Geometry check sheet. Reference: the model listing, model coordinates, mm. A direction names the side the tool comes from. Round coordinates to 2 decimals unless told otherwise and drop trailing zeros. Write each loop counter-clockwise with the first axis right and the second up, starting at its lowest first coordinate (ties: lowest second). Pieces come first, ordered by that corner, then holes. Notation, with made-up numbers: M 47.5,48 L 84.5,48 A23 cw 84.5,60 Z; hole C 30,85.25 d9. An arc over 180 degrees is marked long. One line per item, written item: value. Start each with the question number.
1. Depth check by flat-ended pin: P1, Ø4, axis at x = 9, y = -5.5, coming from the -Z side; P2, Ø2.5, axis at x = 17, y = -5.5, coming from the +Z side; P3, Ø5, axis at y = -4.5, z = -5, coming from the -X side. Enter the tip coordinate at first touch or a pass-through.
2. Scan lines: probe 1 along X at (y, z) = (0.5, -2); probe 2 along Z at (x, y) = (11.5, -6.5); probe 3 along Z at (x, y) = (-3, -7). Record each from-to range of solid material in increasing order. Write a range as [from, to].
3. Release check for a two-part mould opening along X. For faces 4 (the flat face through (19.55, -7, -9)), 5 (the flat face through (13.05, -5, -6)), 6 (the flat face through (18, -7, -7.8)) record: pulls with the +X half, pulls with the -X half, needs draft (parallel to the pull), parting line crosses it, or undercut.
4. Section check D-D (y = -9.5). Record the boundary of the cut face in (x, z).
5. Section check B-B (x = -1.25). Record the boundary of the cut face in (y, z).
6. Access from +Z, -Z, +X, -X, +Y, -Y to the whole of each face (thin tool, end or side, straight path). Record for faces 1 (the flat face through (-2, -2.8, -9)), 2 (the flat face through (1.05, -5, -6)), 3 (the flat face through (16, -5.8, -9)).
7. Section check A-A (z = -9.75). Record the boundary of the cut face in (x, y).
8. Section check C-C (z = -5.25). Record the boundary of the cut face in (x, y).
Autodesk Fusion 360 part; units mm, degrees
sketch "Esquisse1" plane through (0, 0, 0) normal (0, 0, 1) x (1, 0, 0)
  line L0 (0, 0) -> (1.5, 0)
  line L1 (1.5, 0) -> (1.5, 1.2)
  line L2 (1.5, 1.2) -> (0, 1.2)
  line L3 (0, 1.2) -> (0, 0)
  dimension "d1" = 1.5
  dimension "d2" = 1.2
extrude "Extrusion1" add sketch "Esquisse1" along normal blind 1.2
sketch "Esquisse2" plane through (0, 0, 0) normal (0, 0, -1) x (1, 0, 0)
  line L0 (0, 0) -> (0, -1.2)
  line L1 (0, -1.2) -> (1.5, -1.2)
  line L2 (1.5, -1.2) -> (1.5, 0)
  line L3 (1.5, 0) -> (0, 0)
  line L4 (1.35, 0) -> (0.15, 0)
  line L5 (0.15, 0) -> (0.15, -1.2)
  line L6 (0.15, -1.2) -> (1.35, -1.2)
  line L7 (1.35, -1.2) -> (1.35, 0)
  line L8 (0.75, -1.2) -> (0.75, 0)
  dimension "d5" = 1.2
  dimension "d7" = 0.6
extrude "Extrusion2" cut sketch "Esquisse2" against normal blind 1 contours L1 L3 L4 L5 L6 L8 | L1 L3 L4 L6 L7 L8
sketch "Esquisse3" plane through (1.5, 0, 0) normal (1, 0, 0) x (0, 1, 0)
  line L0 (0, 0) -> (1.2, 0)
  line L1 (1.2, 0) -> (1.2, 1.2)
  line L2 (1.2, 1.2) -> (0, 1.2)
  line L3 (0, 1.2) -> (0, 0)
  line L4 (0, 0) -> (0.8, 0)
  line L5 (0.8, 0) -> (0.8, 0.3)
  line L6 (0.8, 0.3) -> (0, 0.3)
  line L7 (0, 0.3) -> (0, 0)
  dimension "d10" = 0.8
  dimension "d11" = 0.3
extrude "Extrusion3" add sketch "Esquisse3" along normal blind 0.5 contours L0 L3 L4 L5 L6 L7
sketch "Esquisse4" plane through (0, 0, 0.3) normal (0, 0, 1) x (-1, 0, 0)
  line L0 (-1.5, -0.8) -> (-1.5, 0)
  line L1 (-1.5, 0) -> (-2, 0)
  line L2 (-2, 0) -> (-2, -0.8)
  line L3 (-2, -0.8) -> (-1.5, -0.8)
  line L4 (-1.5, -0.5) -> (-1.75, -0.5)
  line L5 (-1.75, -0.5) -> (-1.75, -0.3)
  line L6 (-1.75, -0.3) -> (-1.5, -0.3)
  line L7 (-1.5, -0.3) -> (-1.5, -0.5)
  line L8 (-1.5, -0.4) -> (-2, -0.4)
  dimension "d14" = 0.4
  dimension "d15" = 0.1
  dimension "d16" = 0.2
  dimension "d27" = 0.25
extrude "Extrusion4" cut sketch "Esquisse4" against normal blind 0.5 contours L0 L4 L5 L7 L8 | L0 L5 L6 L7 L8
sketch "Esquisse5" plane through (0, 0, 0.3) normal (0, 0, 1) x (-1, 0, 0)
  line L0 (-1.75, -0.3) -> (-1.5, -0.3)
  line L1 (-1.5, -0.3) -> (-1.5, 0)
  line L2 (-1.5, 0) -> (-2, 0)
  line L3 (-2, 0) -> (-2, -0.8)
  line L4 (-2, -0.8) -> (-1.5, -0.8)
  line L5 (-1.5, -0.8) -> (-1.5, -0.5)
  line L6 (-1.5, -0.5) -> (-1.75, -0.5)
  line L7 (-1.75, -0.5) -> (-1.75, -0.3)
sketch "Esquisse6" plane through (0, 0, 0) normal (-1, 0, 0) x (0, -1, 0)
  line L0 (-1.2, 0) -> (0, 0)
  line L1 (0, 0) -> (0, 1.2)
  line L2 (0, 1.2) -> (-1.2, 1.2)
  line L3 (-1.2, 1.2) -> (-1.2, 0)
  line L4 (0, 0) -> (-0.8, 0)
  line L5 (-0.8, 0) -> (-0.8, 0.3)
  line L6 (-0.8, 0.3) -> (0, 0.3)
  line L7 (0, 0.3) -> (0, 0)
  dimension "d19" = 0.8
  dimension "d20" = 0.3
extrude "Extrusion5" add sketch "Esquisse6" along normal blind 0.5 contours L0 L1 L4 L5 L6 L7
sketch "Esquisse7" plane through (0, 0, 0.3) normal (0, 0, 1) x (-1, 0, 0)
  line L0 (0, 0) -> (0, -0.8)
  line L1 (0, -0.8) -> (0.5, -0.8)
  line L2 (0.5, -0.8) -> (0.5, 0)
  line L3 (0.5, 0) -> (0, 0)
  line L4 (0, -0.4) -> (0.5, -0.4)
  line L5 (0, -0.3) -> (0.25, -0.3)
  line L6 (0.25, -0.3) -> (0.25, -0.5)
  line L7 (0.25, -0.5) -> (0, -0.5)
  line L8 (0, -0.5) -> (0, -0.3)
  dimension "d23" = 0.25
  dimension "d24" = 0.2
extrude "Extrusion6" cut sketch "Esquisse7" against normal blind 0.6 contours L0 L4 L5 L6 L8 | L0 L4 L6 L7 L8
fillet "Congé1" radius 0.2 4 edges at (2, 0, 0.15) (2, 0.8, 0.15) (-0.5, 0, 0.15) (-0.5, 0.8, 0.15)
fillet "Congé2" radius 0.05 2 edges at (1.5, 0.6, 1.2) (0, 0.6, 1.2)
fillet "Congé3" radius 0.05 2 edges at (1.35, 0.6, 1) (0.15, 0.6, 1)
scale "Echelle1" factor 10 about (0.05, 1.2, 1.2) bodies 1
Result sheet:
1. P1: stops at z = -0.8
1. P2: stops at z = -7.8
1. P3: stops at x = -0.45
2. probe 1: x = [-0.45, 1.05], [13.05, 14.55]
2. probe 2: z = [-0.8, 1.2]
2. probe 3: z = [-10.8, -7.8]
3. face 4: pulls with the +X half
3. face 5: undercut
3. face 6: needs draft
4. outline: M -5.32,-10.8 L 1.05,-10.8 L 1.05,-1.3 A0.5 cw 1.55,-0.8 L 12.55,-0.8 A0.5 cw 13.05,-1.3 L 13.05,-10.8 L 19.42,-10.8 L 19.42,-7.8 L 14.55,-7.8 L 14.55,0.7 A0.5 ccw 14.05,1.2 L 0.05,1.2 A0.5 ccw -0.45,0.7 L -0.45,-7.8 L -5.32,-7.8 Z
5. outline: M -10.8,-10.8 L -7.8,-10.8 L -7.8,-7.8 L -10.8,-7.8 Z; M -5.8,-10.8 L -2.8,-10.8 L -2.8,-7.8 L -5.8,-7.8 Z
6. face 1: +Z, -Z, -X, +Y
6. face 2: -Z, +Y, -Y
6. face 3: +Z, -Z
7. outline: M -5.45,-8.8 A2 ccw -3.45,-10.8 L 1.05,-10.8 L 1.05,1.2 L -0.45,1.2 L -0.45,-2.8 L -3.45,-2.8 A2 ccw -5.45,-4.8 Z; M 13.05,-10.8 L 17.55,-10.8 A2 ccw 19.55,-8.8 L 19.55,-4.8 A2 ccw 17.55,-2.8 L 14.55,-2.8 L 14.55,1.2 L 13.05,1.2 Z; hole M -2.95,-7.8 L -0.45,-7.8 L -0.45,-5.8 L -2.95,-5.8 Z; hole M 14.55,-7.8 L 17.05,-7.8 L 17.05,-5.8 L 14.55,-5.8 Z
8. outline: M -0.45,-10.8 L 1.05,-10.8 L 1.05,1.2 L -0.45,1.2 Z; M 13.05,-10.8 L 14.55,-10.8 L 14.55,1.2 L 13.05,1.2 Z
